```python
from build123d import *

# Parameters (mm, degrees)
BOSS_EXTRUDE1_DEPTH     = 200
BOSS_EXTRUDE2_DEPTH     = 200
BOSS_EXTRUDE3_START     = 76
SKETCH4_R               = 8.5
BOSS_EXTRUDE3_DEPTH     = 83
BOSS_EXTRUDE4_START     = 48.333333333
BOSS_EXTRUDE4_DEPTH     = 55.333333333
RIB1_START              = -2.5
RIB1_DEPTH              = 5
FILLET3_R               = 10
SKETCH9_R               = 3.5
BOSS_EXTRUDE6_DEPTH     = 50
CUT_EXTRUDE3_DEPTH      = 244.455905202
CUT_EXTRUDE3_DEPTH_BACK = 244.455905202
SKETCH10_R              = 3.5
CUT_EXTRUDE4_DEPTH      = 219.723823831
CUT_EXTRUDE4_DEPTH_BACK = 219.723823831
CUT_EXTRUDE2_DEPTH      = 220.51323992
CUT_EXTRUDE2_DEPTH_BACK = 220.51323992
SKETCH7_R               = 8.5


# Read off the part's stored shape, not the designer's step: Rib1
with BuildPart() as part:
    # Sketch1 → Boss-Extrude1 (new, symmetric)
    with BuildSketch(Plane(origin=(0, 0, 0), x_dir=(1, 0, 0), z_dir=(0, 1, 0))):
        with BuildLine():
            Line((0, 45.75), (4, 45.75))
            Line((4, 45.75), (185.522228719, 14.786424933))
            ThreePointArc((185.522228719, 14.786424933), (198, 0), (185.522228719, -14.786424933))
            Line((185.522228719, -14.786424933), (4, -45.75))
            Line((4, -45.75), (0, -45.75))
            ThreePointArc((0, -45.75), (-45.75, 0), (0, 45.75))
        make_face()
    extrude(amount=BOSS_EXTRUDE1_DEPTH, both=True)


with BuildPart() as body_2:
    # Sketch3 → Boss-Extrude2 (new, symmetric)
    with BuildSketch(Plane.XY):
        Polygon((-45.75, 0), (73.733339697, 0), (138, 45), (198, 45), (198, 52), (135.792908478, 52), (71.526248174, 7), (-45.75, 7), align=None)
    extrude(amount=BOSS_EXTRUDE2_DEPTH, both=True)


with BuildPart() as part_1:
    add(part.part)

    # Combine1: intersect body 2
    add(body_2.part, mode=Mode.INTERSECT)

    # Sketch4 → Boss-Extrude3 (add)
    with BuildSketch(Plane(origin=(0, 7, 0), x_dir=(1, 0, 0), z_dir=(0, 1, 0)).offset(BOSS_EXTRUDE3_START)):
        with BuildLine():
            Line((0, -45.75), (4, -45.75))
            Line((4, -45.75), (4, -11.842719282))
            ThreePointArc((4, -11.842719282), (12.5, 0), (4, 11.842719282))
            Line((4, 11.842719282), (4, 45.75))
            Line((4, 45.75), (0, 45.75))
            ThreePointArc((0, 45.75), (-45.75, 0), (0, -45.75))
        make_face()
        with Locations(Location((0, 0, 0), (0, 0, 270))):
            Circle(SKETCH4_R, mode=Mode.SUBTRACT)
        with BuildLine():
            Line((0, -41.75), (0, -12.5))
            ThreePointArc((0, -12.5), (-12.5, 0), (0, 12.5))
            Line((0, 12.5), (0, 41.75))
            ThreePointArc((0, 41.75), (-41.75, 0), (0, -41.75))
        make_face(mode=Mode.SUBTRACT)
    extrude(amount=-BOSS_EXTRUDE3_DEPTH)

    # Sketch5 → Boss-Extrude4 (add)
    with BuildSketch(Plane(origin=(0, 52, 0), x_dir=(1, 0, 0), z_dir=(0, 1, 0)).offset(BOSS_EXTRUDE4_START)):
        with BuildLine():
            Line((185.522228719, -14.786424933), (183, -14.786424933))
            Line((183, -14.786424933), (183, 14.786424933))
            Line((183, 14.786424933), (185.522228719, 14.786424933))
            ThreePointArc((185.522228719, 14.786424933), (198, 0), (185.522228719, -14.786424933))
        make_face()
        with BuildLine():
            Line((187, -10.246950766), (187, 10.246950766))
            ThreePointArc((187, 10.246950766), (194, 0), (187, -10.246950766))
        make_face(mode=Mode.SUBTRACT)
    extrude(amount=-BOSS_EXTRUDE4_DEPTH)

    # Rib1 outline → Rib1 (add)
    with BuildSketch(Plane.XY.offset(RIB1_START)):
        Polygon((108.349339446, 100.333333333), (83.594773996, 83), (11, 83), (11, 7), (71.526248174, 7), (135.792908478, 52), (183, 52), (183, 100.333333333), align=None)
    extrude(amount=RIB1_DEPTH)

    # Fillet3
    fillet3_edges = [part_1.edges().sort_by_distance(p)[0] for p in [
        (135.792908478, 52, -12.884559521),
        (71.526248174, 7, -18.365776821),
        (108.349339446, 100.333333333, 0),
        (83.594773996, 83, 0),
        (135.792908478, 52, 12.884559521),
        (71.526248174, 7, 18.365776821),
    ]]
    fillet(fillet3_edges, radius=FILLET3_R)

    # Sketch9 → Boss-Extrude6 (add, symmetric)
    with BuildSketch(Plane.XY):
        with BuildLine():
            Line((4, 7), (4, 22))
            Line((4, 22), (39, 22))
            ThreePointArc((39, 22), (46.071067812, 19.071067812), (49, 12))
            Line((49, 12), (49, 7))
            Line((49, 7), (4, 7))
        make_face()
        with Locations((41, 14)):
            Circle(SKETCH9_R, mode=Mode.SUBTRACT)
    extrude(amount=BOSS_EXTRUDE6_DEPTH, both=True)

    # Sketch10 → Cut-Extrude3 (cut, two sides: drawn at the far end of the back side and taken through both)
    with BuildSketch(Plane.XY.offset(50).offset(-CUT_EXTRUDE3_DEPTH_BACK)):
        with Locations((41, 14)):
            Circle(SKETCH10_R)
    extrude(amount=CUT_EXTRUDE3_DEPTH + CUT_EXTRUDE3_DEPTH_BACK, mode=Mode.SUBTRACT)

    # Sketch11 → Cut-Extrude4 (cut, two sides: drawn at the far end of the back side and taken through both)
    with BuildSketch(Plane(origin=(0, 22, 0), x_dir=(1, 0, 0), z_dir=(0, 1, 0)).offset(-CUT_EXTRUDE4_DEPTH_BACK)):
        Polygon((4, -45.75), (49, -38.074020657), (49, -50), (4, -50), align=None)
        Polygon((4, 45.75), (49, 38.074020657), (49, 50), (4, 50), align=None)
    extrude(amount=CUT_EXTRUDE4_DEPTH + CUT_EXTRUDE4_DEPTH_BACK, mode=Mode.SUBTRACT)

    # Sketch7 → Cut-Extrude2 (cut, two sides: drawn at the far end of the back side and taken through both)
    with BuildSketch(Plane(origin=(0, 83, 0), x_dir=(1, 0, 0), z_dir=(0, 1, 0)).offset(-CUT_EXTRUDE2_DEPTH_BACK)):
        with Locations(Location((0, 0, 0), (0, 0, 270))):
            Circle(SKETCH7_R)
        with BuildLine():
            Line((187, 10.246950766), (187, -10.246950766))
            ThreePointArc((187, -10.246950766), (194, 0), (187, 10.246950766))
        make_face()
        with BuildLine():
            Line((0, 12.5), (0, 41.75))
            ThreePointArc((0, 41.75), (-41.75, 0), (0, -41.75))
            Line((0, -41.75), (0, -12.5))
            ThreePointArc((0, -12.5), (-12.5, 0), (0, 12.5))
        make_face()
    extrude(amount=CUT_EXTRUDE2_DEPTH + CUT_EXTRUDE2_DEPTH_BACK, mode=Mode.SUBTRACT)


solid = part_1.part
```
Input: part model. Units: mm. Frame: model coordinates. A direction names the side the tool comes from. Round coordinates to 2 decimals unless told otherwise and drop trailing zeros. Loops run counter-clockwise (first coordinate to the right, second up) from the corner with the lowest first, then second, coordinate; pieces in that order, holes last. Notation, with made-up numbers: M 89.25,30.25 L 114.25,30.25 A26 cw 114.25,69.25 Z; hole C 25,-34.5 d4. An arc over 180 degrees is marked long. Answer in a Markdown table with one row per item. Add a question column.
1. Section D-D (y = 26.5). Output: boundary loops of the cut face in (x, z), and give its area (3 significant figures).
2. Ray query, probe 1 along X at (y, z) = (51, 0); probe 2 along X at (y, z) = (75.5, 2); probe 3 along Z at (x, y) = (-11.5, 76). Return the intervals inside material, ascending.
3. Section B-B (z = 29.5). Output: boundary loops of the cut face in (x, y), and give its area (3 significant figures).
4. Section C-C (y = 70.5). Output: boundary loops of the cut face in (x, z), and give its area (3 significant figures).
5. Set-up query: faces 1 (the face through (108.455, 99.858, 0.035)), 2 (the face through (21, 22, 24)), 3 (the face through (161, 45, 0)), 4 (the face through (49, 10, -20)), 5 (the face through (-12.497, 40.919, 0.275)). Return all of +Z, -Z, +X, -X, +Y, -Y with unobstructed straight access to the full face (end or side cutting, diameter ignored); none if empty.
6. Contact query for flat-ended pins moving along their axis: pin 1 (17.5 mm diameter, centred on x = 22.5, z = 23, fed in from +Y); pin 2 (16.5 mm diameter, centred on y = 63.5, z = -2.5, fed in from +X); pin 3 (15.5 mm diameter, centred on x = 58.5, z = 22.5, fed in from +Y); pin 4 (3 mm diameter, centred on x = 127.5, y = 80, fed in from -Z). Output: stop coordinate, or through.
7. Section A-A (z = 0). Output: boundary loops of the cut face in (x, y).
8. Mould query, pull axis Z, two halves, no side actions, for faces 6 (the face through (0, 41, 27)), 7 (the face through (38.2, 11.9, -0.6)), 8 (the face through (-45.74, 42.08, 1.01)). Classes: released by +Z, released by -Z, zero draft, split by the parting line, or undercut.
Values follow:
| question | item | result |
|---|---|---|
| 1 | outline | M 0,-45.75 L 4,-45.75 L 4,-11.84 A12.5 ccw 12.25,-2.5 L 99.38,-2.5 L 99.38,-29.48 L 111.58,-27.4 L 111.58,27.4 L 99.38,29.48 L 99.38,2.5 L 12.25,2.5 A12.5 ccw 4,11.84 L 4,45.75 L 0,45.75 A45.75 ccw Z; hole C 0,0 d17; hole M 0,-41.75 L 0,-12.5 A12.5 cw 0,12.5 L 0,41.75 A41.75 ccw Z |
| 1 | area | 2,210 mm^2 |
| 2 | probe 1 | -45.75 to -41.75, -12.5 to -8.5, 8.5 to 187, 194 to 198 |
| 2 | probe 2 | -45.71 to -41.7, -12.34 to -8.26, 8.26 to 187, 193.82 to 197.87 |
| 2 | probe 3 | -44.28 to -40.13, -4.9 to 4.9, 40.13 to 44.28 |
| 3 | outline | M -34.97,0 L -29.54,0 L -29.54,83 L -34.97,83 Z; M 0,0 L 73.73,0 L 99.26,17.88 L 99.26,26.42 L 74.11,8.81 A10 cw 68.37,7 L 49,7 L 49,12 A10 ccw 39,22 L 4,22 L 4,83 L 0,83 Z; hole C 41,14 d7 |
| 3 | area | 2,110 mm^2 |
| 4 | outline | M 0,-45.75 L 4,-45.75 L 4,-11.84 A12.5 ccw 12.25,-2.5 L 183,-2.5 L 183,-14.79 L 185.52,-14.79 A15 ccw 185.52,14.79 L 183,14.79 L 183,2.5 L 12.25,2.5 A12.5 ccw 4,11.84 L 4,45.75 L 0,45.75 A45.75 ccw Z; hole C 0,0 d17; hole M 0,-41.75 L 0,-12.5 A12.5 cw 0,12.5 L 0,41.75 A41.75 ccw Z; hole M 187,-10.25 A11 ccw 187,10.25 Z |
| 4 | area | 2,180 mm^2 |
| 5 | face 1 | +Z, -Z, -X, +Y |
| 5 | face 2 | +Z, +Y |
| 5 | face 3 | +Z, -Z, +X, -Y |
| 5 | face 4 | -Z, +Y |
| 5 | face 5 | +Y, -Y |
| 6 | pin 1 | y = 22 |
| 6 | pin 2 | x = 198 |
| 6 | pin 3 | y = 7 |
| 6 | pin 4 | z = -2.5 |
| 7 | outline | M -45.75,0 L -41.75,0 L -41.75,83 L -45.75,83 Z; M -12.5,0 L -8.5,0 L -8.5,83 L -12.5,83 Z; M 8.5,0 L 73.73,0 L 138,45 L 187,45 L 187,100.33 L 111.5,100.33 A10 ccw 105.77,98.52 L 86.18,84.81 A10 cw 80.44,83 L 8.5,83 Z; M 194,45 L 198,45 L 198,100.33 L 194,100.33 Z; hole C 41,14 d7 |
| 8 | face 6 | undercut |
| 8 | face 7 | zero draft |
| 8 | face 8 | split by the parting line |
